Source: CAD feature listing. Evaluate the final solid. Frame: model axes, mm. A direction names the side the tool comes from. Give positions to 0.01 mm unless a question says otherwise; leave off trailing zeros. Order: outer loops, then holes, each group sorted by start corner. A loop starts at its lowest first (then second) coordinate and runs counter-clockwise, first axis right, second up. Notation, with made-up numbers: M 1,-29.75 L 26,-29.75 A25 ccw 26,-12.75 Z; hole C 63,10.25 d8. An arc over 180 degrees is marked long. Use CSV: the item, a comma, the result in double quotes. Start each with the question number.
1. Section query B-B, the plane x = 116. Return the cut outline in (y, z).
2. Line query: line 1 along Y through (x, z) = (122, 130); line 2 along X through (y, z) = (88.5, 130.5); line 3 along Y through (x, z) = (20, 193). Output: solid intervals per line, ascending. Write a range as [from, to].
3. Section query A-A, the plane z = 188.5. Return the cut outline in (x, y).
4. Section query D-D, the plane z = 64. Return the cut outline in (x, y), plus the area to 3 significant figures.
5. Section query C-C, the plane y = 52. Return the cut outline in (x, z), plus the area to 3 significant figures.
6. Mould query, pull axis Y, two halves, no side actions, for faces 4 (the flat face through (65, 24, 225.654)), 5 (the flat face through (65, 41.897, 109)), 6 (the flat face through (65, 171.45, 67)). Classes: released by +Y, released by -Y, zero draft, split by the parting line, or undercut.
7. Reachability of faces 1 (the flat face through (65, 169, 134.976)), 2 (the flat face through (4.763, 106, 67)), 3 (the flat face through (4.763, 23, 109)) from +Z, -Z, +X, -X, +Y, -Y: full face, straight path, thin tool, end or side. Return the list, or none.
from build123d import *

# Parameters (mm, degrees)
SKETCH1_W           = 131.318
SKETCH1_H           = 171.45
BOSS_EXTRUDE1_DEPTH = 134.9756
SKETCH2_W           = 131.318
SKETCH2_H           = 46.6598
BOSS_EXTRUDE2_DEPTH = 90.678
SHELL1_OUTLINE_W    = 121.793
SHELL1_OUTLINE_H    = 161.925
SHELL1_DEPTH        = 134.9756
SHELL1_START        = 134.9756
SHELL1_2_OUTLINE_W  = 121.793
SHELL1_2_OUTLINE_H  = 37.1348
SHELL1_2_DEPTH      = 85.9155
SKETCH3_W           = 131.318
SKETCH3_H           = 134.9756
BOSS_EXTRUDE3_DEPTH = 4.7625


# Read off the part's stored shape, not the designer's step: Shell1
with BuildPart() as part:
    # Sketch1 → Boss-Extrude1 (new body)
    with BuildSketch(Plane.XY):
        with Locations((65.659, 85.725)):
            Rectangle(SKETCH1_W, SKETCH1_H)
    extrude(amount=BOSS_EXTRUDE1_DEPTH)

    # Sketch2 → Boss-Extrude2 (add)
    with BuildSketch(Plane.XY.offset(134.9756)):
        with Locations((65.659, 23.3299)):
            Rectangle(SKETCH2_W, SKETCH2_H)
    extrude(amount=BOSS_EXTRUDE2_DEPTH)

    # Shell1 outline → Shell1 (cut)
    with BuildSketch(Plane.XY):
        with Locations((65.659, 85.725)):
            Rectangle(SHELL1_OUTLINE_W, SHELL1_OUTLINE_H)
    extrude(amount=SHELL1_DEPTH, mode=Mode.SUBTRACT)

    # Shell1 2 outline → Shell1 2 (cut)
    with BuildSketch(Plane.XY.offset(SHELL1_START)):
        with Locations((65.659, 23.3299)):
            Rectangle(SHELL1_2_OUTLINE_W, SHELL1_2_OUTLINE_H)
    extrude(amount=SHELL1_2_DEPTH, mode=Mode.SUBTRACT)

    # Sketch3 → Boss-Extrude3 (add)
    with BuildSketch(Plane(origin=(0, 46.6598, 0), x_dir=(1, 0, 0), z_dir=(0, 1, 0))):
        with Locations((65.659, -67.4878)):
            Rectangle(SKETCH3_W, SKETCH3_H)
    extrude(amount=-BOSS_EXTRUDE3_DEPTH)


solid = part.part
Result set:
1,outline,"M 0,0 L 4.76,0 L 4.76,220.89 L 41.9,220.89 L 41.9,0 L 46.66,0 L 46.66,225.65 L 0,225.65 Z; M 166.69,0 L 171.45,0 L 171.45,134.98 L 166.69,134.98 Z"
2,line 1,"[0, 4.76], [41.9, 46.66], [166.69, 171.45]"
2,line 2,"[0, 4.76], [126.56, 131.32]"
2,line 3,"[0, 4.76], [41.9, 46.66]"
3,outline,"M 0,0 L 131.32,0 L 131.32,46.66 L 0,46.66 Z; hole M 4.76,4.76 L 126.56,4.76 L 126.56,41.9 L 4.76,41.9 Z"
4,outline,"M 0,0 L 131.32,0 L 131.32,171.45 L 0,171.45 Z; hole M 4.76,4.76 L 126.56,4.76 L 126.56,41.9 L 4.76,41.9 Z; hole M 4.76,46.66 L 126.56,46.66 L 126.56,166.69 L 4.76,166.69 Z"
4,area,"3,370 mm2"
5,outline,"M 0,0 L 4.76,0 L 4.76,134.98 L 0,134.98 Z; M 126.56,0 L 131.32,0 L 131.32,134.98 L 126.56,134.98 Z"
5,area,"1,290 mm2"
6,face 4,"zero draft"
6,face 5,"undercut"
6,face 6,"released by +Y"
7,face 1,"+Z, +X, -X, +Y"
7,face 2,"+Z, -Z"
7,face 3,"-Z"
